Read the model definition and answer for the solid it produces. Units are mm, in the model's axes. Face numbers are marked on the shaded views. A direction names the side the tool comes from. Coordinates: 2 decimals unless noted, no trailing zeros. Order: outer loops, then holes, each group sorted by start corner. A loop starts at its lowest first (then second) coordinate and runs counter-clockwise, first axis right, second up. Notation, with made-up numbers: (41.5, 37) - (51.5, 37) arc R31 ccw to (51.5, 71) - close; hole circle Ø1 at (29, 63). An arc over 180 degrees is marked (long way). Write item = value, one per line.
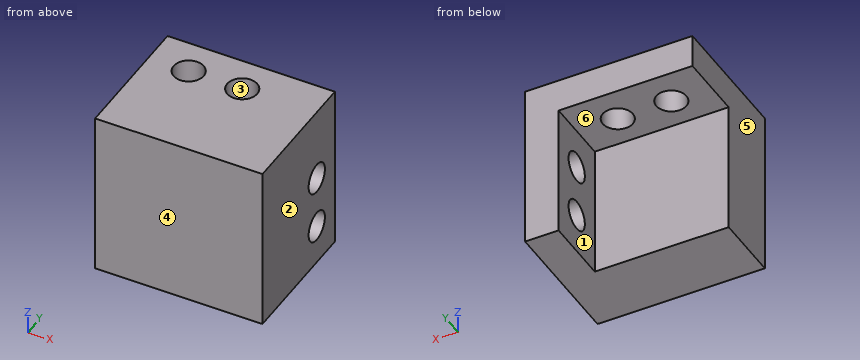
Autodesk Inventor part; units mm, degrees
ref_plane "YZ Plane" through (0, 0, 0) normal (1, 0, 0) x (0, 1, 0)
ref_plane "XZ Plane" through (0, 0, 0) normal (0, 1, 0) x (-1, 0, 0)
ref_plane "XY Plane" through (0, 0, 0) normal (0, 0, 1) x (1, 0, 0)
sketch "Sketch1" plane through (0, 0, 0) normal (0, 0, 1) x (1, 0, 0)
  line L0 (-12.5, -10) -> (12.5, -10)
  line L1 (12.5, -10) -> (12.5, 10)
  line L2 (12.5, 10) -> (-12.5, 10)
  line L3 (-12.5, 10) -> (-12.5, -10)
  line L4 (-12.5, -10) -> (12.5, 10) construction
  line L5 (12.5, -10) -> (-12.5, 10) construction
  point P0 (0, 0)
  dimension "d0" = 25
  dimension "d1" = 20
extrude "Extrusion1" add sketch "Sketch1" along normal blind 25
sketch "Sketch2" plane through (-12.5, 10, 0) normal (0, 1, 0) x (1, 0, 0)
  line L0 (0, 0) -> (25, 0)
  line L1 (0, 0) -> (20, 0)
  line L2 (20, 0) -> (20, -20)
  line L3 (20, -20) -> (0, -20)
  line L4 (0, -20) -> (0, 0)
  point P0 (12.5, 0)
  point P1 (20, 0)
  dimension "d4" = 20
  dimension "d5" = 20
extrude "Extrusion2" cut sketch "Sketch2" against normal blind 10
sketch "Sketch3" plane through (7.5, 10, 0) normal (-1, 0, 0) x (0, 0, 1)
  circle A0 centre (6, -5) radius 2.25
  circle A1 centre (14, -5) radius 2.25
  line L0 (0, 0) -> (20, 0)
  line L1 (20, -10) -> (0, -10)
  line L2 (0, -10) -> (0, 0)
  line L3 (20, 0) -> (20, -10)
  dimension "d8" = 4.5
  dimension "d9" = 4.5
  dimension "d10" = 5
  dimension "d11" = 10
  dimension "d12" = 5
  dimension "d14" = 20
  dimension "d17" = 8
  dimension "d18" = 6
extrude "Extrusion3" cut sketch "Sketch3" against normal blind 5 contours A0 | A1
thread "Thread1"
thread "Thread2"
sketch "Sketch4" plane through (7.5, 10, 20) normal (0, 0, -1) x (-1, 0, 0)
  circle A0 centre (6, -5.25) radius 2.25
  circle A1 centre (14, -5.25) radius 2.25
  line L0 (0, 0) -> (20, 0)
  line L1 (20, 0) -> (20, -10)
  line L2 (0, 0) -> (0, -10)
  point P0 (7.5, -10)
  dimension "d25" = 4.5
  dimension "d26" = 4.5
  dimension "d27" = 8
  dimension "d28" = 3
  dimension "d29" = 3
  dimension "d30" = 6
  dimension "d31" = 6
extrude "Extrusion4" cut sketch "Sketch4" against normal blind 5
thread "Thread3"
thread "Thread4"
properties part number "CONTOL_COMBI"
1) Flat-ended cylindrical pins translate along their axes: pin 1 Ø4 at (x, y) = (0, 5) entering from -Z; pin 2 Ø8 at (y, z) = (5.5, 15) entering from -X; pin 3 Ø6 at (x, z) = (-6, 12) entering from +Y. Find the tip coordinate at first contact, or state that the pin passes through.
Returned:
pin_1 = 20
pin_2 = 7.5
pin_3 = 0
2) The part is cut by section B-B (x = 1.5). Determine the outline of the cut face in (y, z), and give its area (4 significant figures).
Returned:
outline = (-10, 0) - (0, 0) - (0, 20) - (2.5, 20) - (2.5, 25) - (-10, 25) - close; (7, 20) - (10, 20) - (10, 25) - (7, 25) - close
area = 277.5 mm^2
3) The part is cut by section D-D (y = 4). Determine the outline of the cut face in (x, z).
Returned:
outline = (-12.5, 20) - (-8.62, 20) - (-8.62, 25) - (-12.5, 25) - close; (-4.38, 20) - (-0.62, 20) - (-0.62, 25) - (-4.38, 25) - close; (3.62, 20) - (7.5, 20) - (7.5, 16.02) - (12.5, 16.02) - (12.5, 25) - (3.62, 25) - close; (7.5, 0) - (12.5, 0) - (12.5, 3.98) - (7.5, 3.98) - close; (7.5, 8.02) - (12.5, 8.02) - (12.5, 11.98) - (7.5, 11.98) - close
4) For the marked faces 5 and 6, determine the directions among +Z, -Z, +X, -X, +Y, -Y from which every point of the face is accessible in a straight line to the end or side of a thin tool.
Returned:
face_5 = +Z, -Z, -X, +Y, -Y
face_6 = -Z, -X, +Y
5) The part is cut by section A-A (z = 14). Determine the outline of the cut face in (x, y), and give its area (4 significant figures).
Returned:
outline = (-12.5, -10) - (12.5, -10) - (12.5, 2.75) - (7.5, 2.75) - (7.5, 0) - (-12.5, 0) - close; (7.5, 7.25) - (12.5, 7.25) - (12.5, 10) - (7.5, 10) - close
area = 277.5 mm^2
6) Straight lines are drawn through the part: line 1 along Y through (x, z) = (8.85, 14); line 2 along Y through (x, z) = (-6.5, 23.8); line 3 along Y through (x, z) = (-10, 11). For each, find the intervals that lie inside material, in ascending order. Write a range as from..to.
Returned:
line_1 = -10..2.75, 7.25..10
line_2 = -10..2.5, 7..10
line_3 = -10..0
7) Determine the mould class of the marked faces 1, 2, 3 and 4 for opening direction X: pulls with the +X half, pulls with the -X half, needs draft (parallel to the pull), parting line crosses it, or undercut.
Returned:
face_1 = pulls with the -X half
face_2 = pulls with the +X half
face_3 = undercut
face_4 = needs draft
8) The part is cut by section C-C (x = 9.5). Determine the outline of the cut face in (y, z).
Returned:
outline = (-10, 0) - (10, 0) - (10, 25) - (-10, 25) - close; hole circle Ø4.5 at (5, 6); hole circle Ø4.5 at (5, 14)
